Could you check a few things on this model? Use its own coordinates, in mm. A direction names the side the tool comes from. Give positions to 0.01 mm unless a question says otherwise; leave off trailing zeros. Write each loop counter-clockwise with the first axis right and the second up, starting at its lowest first coordinate (ties: lowest second). Pieces come first, ordered by that corner, then holes. Notation, with made-up numbers: M -2,77 L 47,77 A24 ccw 47,112 Z; hole C 71.25,50.5 d3. An arc over 180 degrees is marked long. One line per item, written item: value.
```python
from build123d import *

# Parameters (mm, degrees)
SKETCH1_R           = 12.5
BOSS_EXTRUDE1_DEPTH = 1.5
SKETCH2_R           = 11
BOSS_EXTRUDE2_DEPTH = 7
SKETCH3_R           = 4
CUT_EXTRUDE1_DEPTH  = 20.615045246
SKETCH4_R           = 9.5
SKETCH4_R_2         = 5.5
CUT_EXTRUDE2_DEPTH  = 0.08
CUT_EXTRUDE3_START  = -0.08
SKETCH5_R           = 9.5
SKETCH5_R_2         = 5.5
CUT_EXTRUDE3_DEPTH  = 0.08
FILLET1_R           = 0.31


with BuildPart() as part:
    # Sketch1 → Boss-Extrude1 (new body)
    with BuildSketch(Plane(origin=(0, 0, 0), x_dir=(1, 0, 0), z_dir=(0, 1, 0))):
        with Locations(Location((0, 0, 0), (0, 0, 270))):
            Circle(SKETCH1_R)
    extrude(amount=BOSS_EXTRUDE1_DEPTH)

    # Sketch2 → Boss-Extrude2 (add)
    with BuildSketch(Plane(origin=(0, 1.5, 0), x_dir=(1, 0, 0), z_dir=(0, 1, 0))):
        with Locations(Location((0, 0, 0), (0, 0, 270))):
            Circle(SKETCH2_R)
    extrude(amount=BOSS_EXTRUDE2_DEPTH)

    # Sketch3 → Cut-Extrude1 (cut, through all)
    with BuildSketch(Plane(origin=(0, 8.5, 0), x_dir=(1, 0, 0), z_dir=(0, 1, 0))):
        with Locations(Location((0, 0, 0), (0, 0, 270))):
            Circle(SKETCH3_R)
    extrude(amount=-CUT_EXTRUDE1_DEPTH, mode=Mode.SUBTRACT)

    # Sketch4 → Cut-Extrude2 (cut)
    with BuildSketch(Plane.XZ):
        with Locations(Location((0, 0, 0), (0, 0, 270))):
            Circle(SKETCH4_R)
        with Locations(Location((0, 0, 0), (0, 0, 270))):
            Circle(SKETCH4_R_2, mode=Mode.SUBTRACT)
    extrude(amount=-CUT_EXTRUDE2_DEPTH, mode=Mode.SUBTRACT)

    # Sketch5 → Cut-Extrude3 (cut)
    with BuildSketch(Plane(origin=(0, 8.5, 0), x_dir=(1, 0, 0), z_dir=(0, 1, 0)).offset(CUT_EXTRUDE3_START)):
        with Locations(Location((0, 0, 0), (0, 0, 90))):
            Circle(SKETCH5_R)
        with Locations(Location((0, 0, 0), (0, 0, 90))):
            Circle(SKETCH5_R_2, mode=Mode.SUBTRACT)
    extrude(amount=CUT_EXTRUDE3_DEPTH, mode=Mode.SUBTRACT)

    # Fillet1
    fillet1_edges = [part.edges().sort_by_distance(p)[0] for p in [
        (0, 0, -4),
        (0, 8.5, -4),
        (0, 0, -12.5),
        (0, 1.5, -12.5),
        (0, 8.5, -11),
    ]]
    fillet(fillet1_edges, radius=FILLET1_R)


solid = part.part
```
1) Please list where these lines run through material, in increasing order: L1, parallel to X at y = 5.25, z = 0; L2, parallel to Y at x = 6.5, z = 3.75; L3, parallel to X at y = 5.25, z = -0.75. Write a range as from..to.
Outcome:
L1: x = -11..-4, 4..11
L2: y = 0.08..8.42
L3: x = -10.97..-3.93, 3.93..10.97
2) I'm going to push flat-ended pins straight in: pin 1 (4 mm diameter, centred on x = 0, y = 2, fed in from -Z); pin 2 (1.5 mm diameter, centred on y = 5.5, z = 5.5, fed in from +X); pin 3 (1.5 mm diameter, centred on y = 1.5, z = -2.5, fed in from -X); pin 4 (5 mm diameter, centred on x = 6, y = 1.5, fed in from +Z). Where does each tip first touch, or does it pass through?
Outcome:
pin 1: stops at z = -12.5
pin 2: stops at x = 9.92
pin 3: stops at x = -12.37
pin 4: stops at z = 11.99
3) If we section it at A-A, the plane y = 3.5: Write out the boundary of the cut face in (x, z), then the cut area to 3 significant figures.
Outcome:
outline: C 0,0 d22; hole C 0,0 d8
area: 330 mm^2
4) We'd pull the mould along X, two halves only. Please class faces 1 (the face through (11, 1.5, -2)), 2 (the face through (3.755, 0.744, 11.923)), 3 (the face through (-3.905, 4.305, -0.867)): pulls with the +X half, pulls with the -X half, needs draft (parallel to the pull), parting line crosses it, or undercut.
Outcome:
face 1: needs draft
face 2: parting line crosses it
face 3: undercut
5) On a 3-axis mill with a long thin cutter (end or side, diameter ignored), from which of +Z, -Z, +X, -X, +Y, -Y can I reach the whole of each face in a straight line? I mean faces 4 (the face through (10, 8.5, 0)), 5 (the face through (-10.74, 4.8, -2.38)), 6 (the face through (-4, 0.08, -4)). Say none if no direction works.
Outcome:
face 4: +Z, -Z, +X, -X, +Y
face 5: +Y
face 6: -Y
